Geometry: see drawing. Coordinates: mm, zero at the bounding-box minimum. A direction names the side the tool comes from. Round coordinates to 2 decimals unless told otherwise and drop trailing zeros. Write each loop counter-clockwise with the first axis right and the second up, starting at its lowest first coordinate (ties: lowest second). Pieces come first, ordered by that corner, then holes. Notation, with made-up numbers: (14.5, 50) - (43.5, 50) arc R26 cw to (43.5, 81) - close; hole circle Ø1 at (10.25, 77). An arc over 180 degrees is marked (long way). One line per item, written item: value. Start each with the question number.
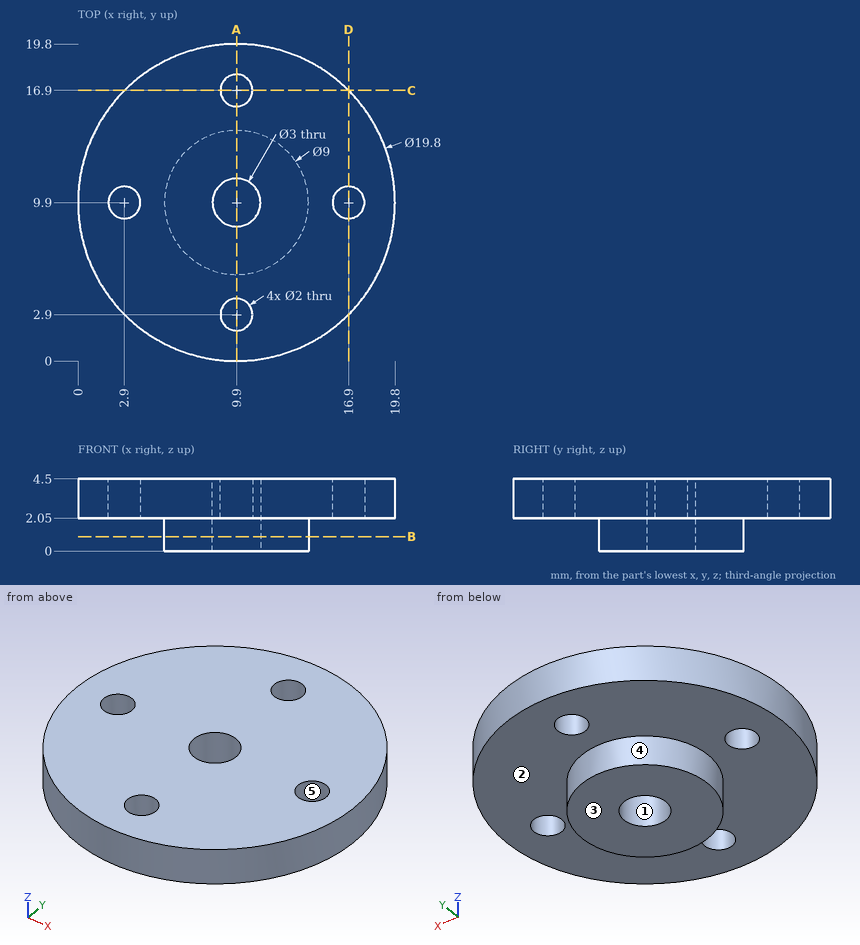
Q1. Cut plane B-B, the plane z = 0.9. Output: boundary loops of the cut face in (x, y), and give its area (3 significant figures).
Q2. Contact query for flat-ended pins moving along their axis: pin 1 Ø1 at (y, z) = (14.5, 3) entering from -X; pin 2 Ø1.2 at (x, y) = (2.9, 9.9) entering from -Z; pin 3 Ø2 at (x, z) = (5, 4) entering from -Y. Output: stop coordinate, or through.
Q3. Access query for the marked faces 1 and 2. Directions: +Z, -Z, +X, -X, +Y, -Y. A direction counts if a zero-diameter tool reaches every point of the face in a straight line with its end or side. Return the directions, or none.
Q4. Cut plane A-A, the plane x = 9.9. Output: boundary loops of the cut face in (y, z), and give its area (3 significant figures).
Q5. Cut plane C-C, the plane y = 16.9. Output: boundary loops of the cut face in (x, z).
Q6. Pull-direction query (Y, two-part tool) for the marked faces 3, 4 and 5; classes: pulls with the +Y half, pulls with the -Y half, needs draft (parallel to the pull), parting line crosses it, or undercut.
Q7. Material intervals for probe 1 along Y at (x, z) = (9.9, 3.4); probe 2 along X at (y, z) = (10.25, 3.4); probe 3 along Z at (x, y) = (18.5, 11.5), sorted ascending. Write a range as from..to.
A:
1. outline: circle Ø9 at (9.9, 9.9); hole circle Ø3 at (9.9, 9.9)
1. area: 56.5 mm²
2. pin 1: stops at x = 0.89
2. pin 2: passes through
2. pin 3: stops at y = 0.8
3. face 1: +Z, -Z
3. face 2: -Z
4. outline: (0, 2.05) - (1.9, 2.05) - (1.9, 4.5) - (0, 4.5) - close; (3.9, 2.05) - (5.4, 2.05) - (5.4, 0) - (8.4, 0) - (8.4, 4.5) - (3.9, 4.5) - close; (11.4, 0) - (14.4, 0) - (14.4, 2.05) - (15.9, 2.05) - (15.9, 4.5) - (11.4, 4.5) - close; (17.9, 2.05) - (19.8, 2.05) - (19.8, 4.5) - (17.9, 4.5) - close
4. area: 43.7 mm²
5. outline: (2.9, 2.05) - (8.9, 2.05) - (8.9, 4.5) - (2.9, 4.5) - close; (10.9, 2.05) - (16.9, 2.05) - (16.9, 4.5) - (10.9, 4.5) - close
6. face 3: needs draft
6. face 4: parting line crosses it
6. face 5: undercut
7. probe 1: y = 0..1.9, 3.9..8.4, 11.4..15.9, 17.9..19.8
7. probe 2: x = 0.01..1.96, 3.84..8.44, 11.36..15.96, 17.84..19.79
7. probe 3: z = 2.05..4.5
